Autodesk Inventor part; units mm, degrees
ref_plane "Work Plane1" through (90, 0, 0) normal (-1, 0, 0) x (0, 0, 1)
ref_plane "Work Plane2" through (0, -15, 0) normal (0, 1, 0) x (-1, 0, 0)
ref_plane "YZ Plane" through (0, 0, 0) normal (1, 0, 0) x (0, 1, 0)
sketch "Sketch1" plane through (0, 0, 0) normal (1, 0, 0) x (0, 1, 0)
  circle A0 centre (0, 0) radius 15
  circle A1 centre (0, 0) radius 13
  dimension "d0" = 30
  dimension "d1" = 26
extrude "Extrusion1" add sketch "Sketch1" along normal blind 180
sketch "Sketch2" plane through (0, 0, 0) normal (0, 1, 0) x (-1, 0, 0)
  line L0 (0, 0) -> (-180, 0) construction
  line L1 (-180, 15) -> (-180, -15) construction
  line L2 (-11, 2) -> (0, 2)
  line L3 (0, 2) -> (0, -2)
  line L4 (0, -2) -> (-11, -2)
  line L5 (-11, -2) -> (-11, 2)
  line L6 (-11, 2) -> (0, -2)
  line L7 (0, 2) -> (-11, -2)
  line L8 (0, -15) -> (0, 15)
  line L9 (0, 15) -> (0, -15)
  line L10 (0, -15) -> (-180, -15)
  point P0 (-5.5, 0)
  dimension "d4" = 4
  dimension "d5" = 11
extrude "Extrusion2" cut sketch "Sketch2" against normal through all
fillet "Fillet1" radius 2 2 edges at (11, -13.8557, 2) (11, -13.8557, -2)
ref_plane "Work Plane1" through (90, 0, 0) normal (-1, 0, 0) x (0, 0, 1)
mirror "Mirror1" about plane through (90, 0, 0) normal (-1, 0, 0) of "Extrusion2", "Fillet1"
ref_plane "Work Plane2" through (0, -15, 0) normal (0, 1, 0) x (-1, 0, 0)
properties part number "Laser_tube" material "Polycarbonate, Clear"
Geometry check sheet. Reference: the model listing, model coordinates, mm. Coordinates: 2 decimals unless noted, no trailing zeros. Order: outer loops, then holes, each group sorted by start corner. A loop starts at its lowest first (then second) coordinate and runs counter-clockwise, first axis right, second up.
Item 1: Section check A-A (y = 0). Enter the section's corners in (x, z), plus the area to 3 significant figures.
Item 2: Mould release check, pull along Z, two halves, no side actions. Record for faces 1 (the cylindrical face through (88.74, 14.307, -4.506)), 2 (the flat face through (180, 6, -12)), 3 (the cylindrical face through (88.7, 12.4, -3.9)): released by +Z, released by -Z, zero draft, split by the parting line, or undercut.
Item 3: Scan lines: line 1 along Y through (x, z) = (116, 0); line 2 along Z through (x, y) = (28.5, 6). Record each from-to range of solid material in increasing order.
Item 4: Section check B-B (x = 30). Enter the section's corners in (y, z), plus the area to 3 significant figures.
Item 5: Depth check by flat-ended pin: pin 1 (1.6 mm diameter, centred on x = 5.5, y = -13.5, fed in from -Z); pin 2 (6 mm diameter, centred on y = 4, z = -11, fed in from +X); pin 3 (10 mm diameter, centred on x = 95.5, z = 9, fed in from +Y); pin 4 (1.5 mm diameter, centred on x = 40.5, z = -9, fed in from +Y). Enter the tip coordinate at first touch or a pass-through.
Item 6: Section check C-C (y = -6.5). Enter the section's corners in (x, z), plus the area to 3 significant figures.
Check sheet entries:
1. outline: (0, -15) - (180, -15) - (180, -13) - (0, -13) - close; (0, 13) - (180, 13) - (180, 15) - (0, 15) - close
1. area: 720 mm2
2. face 1: split by the parting line
2. face 2: zero draft
2. face 3: undercut
3. line 1: y = -15 to -13, 13 to 15
3. line 2: z = -13.75 to -11.53, 11.53 to 13.75
4. outline: circle Ø30 at (0, 0); hole circle Ø26 at (0, 0)
4. area: 176 mm2
5. pin 1: stops at z = -7.98
5. pin 2: stops at x = 180
5. pin 3: stops at y = 14.46
5. pin 4: stops at y = 12.53
6. outline: (0, -13.52) - (180, -13.52) - (180, -11.26) - (0, -11.26) - close; (0, 11.26) - (180, 11.26) - (180, 13.52) - (0, 13.52) - close
6. area: 814 mm2
